For this review, use the dimensioned drawing (mm, ordinates from the lowest corner) and the shaded views. Give positions to 0.01 mm unless a question says otherwise; leave off trailing zeros. Loops run counter-clockwise (first coordinate to the right, second up) from the corner with the lowest first, then second, coordinate; pieces in that order, holes last. Notation, with made-up numbers: (-14.5, -39.5) - (-3.5, -39.5) arc R9 ccw to (-3.5, -23.5) - close; hole circle Ø9 at (62.5, 7). An arc over 180 degrees is marked (long way). Put each result on its own line as item: value.
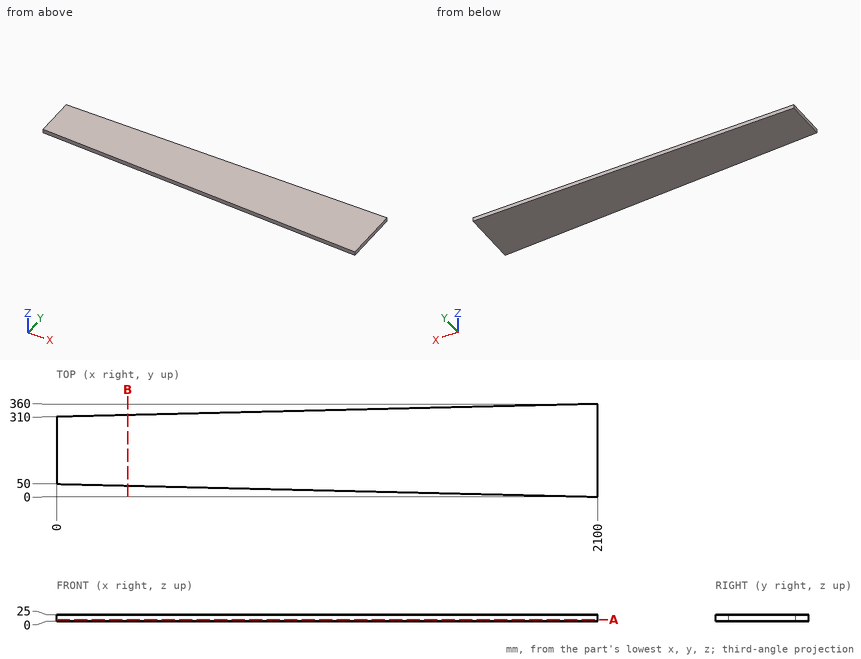
1) Wall thickness on line 1 (Y direction, x = 806, z = 7.75); line 2 (Y direction, x = 1843, z = 13): over which ranges is each line inside the solid? List them lowest first.
Geometry check:
line 1: y = 30.81 to 329.19
line 2: y = 6.12 to 353.88
2) Take a section at A-A on z = 5.75. State the section outline as (x, y) points.
Geometry check:
outline: (0, 50) - (2100, 0) - (2100, 360) - (0, 310) - close
3) Insertion check: pin 1 Ø4 at (x, z) = (1641.5, 9) entering from -Y; pin 2 Ø5 at (x, z) = (1424, 17) entering from -Y; pin 3 Ø10 at (x, z) = (308.5, 8) entering from -Y; pin 4 Ø12 at (y, z) = (99.5, 14.5) entering from -X. Each pin has a flat end and moves straight along its axis. Give the tip position at first contact, or say it passes through.
Geometry check:
pin 1: stops at y = 10.87
pin 2: stops at y = 16.04
pin 3: stops at y = 42.54
pin 4: stops at x = 0
4) Take a section at B-B on x = 275.5. State the section outline as (y, z) points.
Geometry check:
outline: (43.44, 0) - (316.56, 0) - (316.56, 25) - (43.44, 25) - close
